Work out the finished part from the listing and answer in its coordinate system (mm). A direction names the side the tool comes from. Give positions to 0.01 mm unless a question says otherwise; leave off trailing zeros. Order: outer loops, then holes, each group sorted by start corner. A loop starts at its lowest first (then second) coordinate and runs counter-clockwise, first axis right, second up. Notation, with made-up numbers: (67.25, -8) - (75.25, -8) arc R21 ccw to (75.25, 16) - close; hole circle Ø2 at (50, -15.5). An arc over 180 degrees is marked (long way). Put each result on its own line as item: value.
```python
from build123d import *

# Parameters (mm, degrees)
SKETCH1_W           = 45
SKETCH1_H           = 15
SKETCH1_R           = 1
BOSS_EXTRUDE1_DEPTH = 0.5
SKETCH2_W           = 10
SKETCH2_H           = 3.5
BOSS_EXTRUDE2_DEPTH = 10
SKETCH3_W           = 3.374290432
SKETCH3_H           = 2.788954337
SKETCH3_W_2         = 1.377261401
SKETCH3_H_2         = 5.956655559
SKETCH3_H_3         = 1.10180912
SKETCH3_W_3         = 1.790439821
SKETCH3_H_4         = 5.922224024
BOSS_EXTRUDE3_DEPTH = 2


with BuildPart() as part:
    # Sketch1 → Boss-Extrude1 (new, symmetric)
    with BuildSketch(Plane(origin=(0, 0, 0), x_dir=(1, 0, 0), z_dir=(0, 1, 0))):
        Rectangle(SKETCH1_W, SKETCH1_H)
        with Locations(Location((-20.5, 5.5, 0), (0, 0, 270))):
            Circle(SKETCH1_R, mode=Mode.SUBTRACT)
        with Locations(Location((20.5, -5.5, 0), (0, 0, 270))):
            Circle(SKETCH1_R, mode=Mode.SUBTRACT)
    extrude(amount=BOSS_EXTRUDE1_DEPTH, both=True)

    # Sketch2 → Boss-Extrude2 (add)
    with BuildSketch(Plane(origin=(0, 0.5, 0), x_dir=(1, 0, 0), z_dir=(0, 1, 0))):
        with Locations((-10.5, 4.75)):
            Rectangle(SKETCH2_W, SKETCH2_H)
        with Locations((5.5, 4.75)):
            Rectangle(SKETCH2_W, SKETCH2_H)
    extrude(amount=BOSS_EXTRUDE2_DEPTH)

    # Sketch3 → Boss-Extrude3 (add)
    with BuildSketch(Plane(origin=(0, 0.5, 0), x_dir=(1, 0, 0), z_dir=(0, 1, 0))):
        with Locations((-1.687145216, 1.394477169)):
            Rectangle(SKETCH3_W, SKETCH3_H)
        with Locations((-20.176879524, -2.97832778)):
            Rectangle(SKETCH3_W_2, SKETCH3_H_2)
        with Locations((-1.687145216, -5.956655559)):
            Rectangle(SKETCH3_W, SKETCH3_H_3)
        with Locations((19.970290314, 1.756008286)):
            Rectangle(SKETCH3_W_3, SKETCH3_H_4)
    extrude(amount=BOSS_EXTRUDE3_DEPTH)


solid = part.part
```
(1) Section B-B, the plane y = 9.5 is taken. Write down the section's boundary in (x, z), then the cut area to 3 significant figures.
Geometry check:
outline: (-15.5, -6.5) - (-5.5, -6.5) - (-5.5, -3) - (-15.5, -3) - close; (0.5, -6.5) - (10.5, -6.5) - (10.5, -3) - (0.5, -3) - close
area: 70.0 mm²
(2) Section A-A, the plane z = -5.5 is taken. Write down the section's boundary in (x, y), then the cut area to 3 significant figures.
Geometry check:
outline: (-22.5, -0.5) - (-21.5, -0.5) - (-21.5, 0.5) - (-22.5, 0.5) - close; (-19.5, -0.5) - (22.5, -0.5) - (22.5, 0.5) - (10.5, 0.5) - (10.5, 10.5) - (0.5, 10.5) - (0.5, 0.5) - (-5.5, 0.5) - (-5.5, 10.5) - (-15.5, 10.5) - (-15.5, 0.5) - (-19.5, 0.5) - close
area: 243 mm²
(3) Given pin 1 (3 mm diameter, centred on x = -11.5, y = 5, fed in from -Z); pin 2 (6 mm diameter, centred on y = 7, z = -1.5, fed in from +X); pin 3 (1.2 mm diameter, centred on y = 2, z = 6, fed in from +X), each flat-ended and moving along its own axis, determine where each tip first touches the part or whether it passes through.
Geometry check:
pin 1: stops at z = -6.5
pin 2: stops at x = 10.5
pin 3: stops at x = 0
(4) Straight lines are drawn through the part: line 1 (X direction, y = 0.05, z = -5.5); line 2 (X direction, y = 0.15, z = 5.5); line 3 (Y direction, x = 4, z = 5). For each, find the intervals that lie inside material, in ascending order.
Geometry check:
line 1: x = -22.5 to -21.5, -19.5 to 22.5
line 2: x = -22.5 to 19.5, 21.5 to 22.5
line 3: y = -0.5 to 0.5
(5) Determine the mould class of faces 1 (the face through (-22.5, 0, 0)), 2 (the face through (-3.374, 1, 6)), 3 (the face through (20.866, 1, -2)) for opening direction X: pulls with the +X half, pulls with the -X half, needs draft (parallel to the pull), parting line crosses it, or undercut.
Geometry check:
face 1: pulls with the -X half
face 2: undercut
face 3: pulls with the +X half
(6) Section C-C, the plane x = -2 is taken. Write down the section's boundary in (y, z).
Geometry check:
outline: (-0.5, -7.5) - (0.5, -7.5) - (0.5, -2.79) - (2.5, -2.79) - (2.5, 0) - (0.5, 0) - (0.5, 5.41) - (2.5, 5.41) - (2.5, 6.51) - (0.5, 6.51) - (0.5, 7.5) - (-0.5, 7.5) - close
(7) Section D-D, the plane z = 2.25 is taken. Write down the section's boundary in (x, y), then the cut area to 3 significant figures.
Geometry check:
outline: (-22.5, -0.5) - (22.5, -0.5) - (22.5, 0.5) - (-19.49, 0.5) - (-19.49, 2.5) - (-20.87, 2.5) - (-20.87, 0.5) - (-22.5, 0.5) - close
area: 47.8 mm²
(8) A tool of negligible diameter and unlimited length cuts with its end or side. For faces 4 (the face through (-2, 1, -2.789)), 5 (the face through (20, 2.5, -2)), 6 (the face through (-11, 5, -6.5)), 7 (the face through (-5.5, 5, -5)), from which of +Z, -Z, +X, -X, +Y, -Y can it reach the whole face along a straight path? Write none if from no direction.
Geometry check:
face 4: -Z, -X, +Y
face 5: +Z, -Z, +X, +Y
face 6: -Z, +X, -X, +Y
face 7: +Z, -Z, +Y
